Can you work these out from the model? Positions are in its coordinate system, mm. A direction names the side the tool comes from. Coordinates: 2 decimals unless noted, no trailing zeros. Loops run counter-clockwise (first coordinate to the right, second up) from the corner with the lowest first, then second, coordinate; pieces in that order, holes last.
```python
from build123d import *

# Parameters (mm, degrees)
CROQUIS1_W              = 20
CROQUIS1_H              = 72.5
CROQUIS1_R              = 1.6
SALIENTE_EXTRUIR1_DEPTH = 5
CORTAR_EXTRUIR1_DEPTH   = 2
CROQUIS3_W              = 20
CROQUIS3_H              = 8
SALIENTE_EXTRUIR2_DEPTH = 45
CROQUIS4_R              = 2.25
CROQUIS4_R_2            = 3
CORTAR_EXTRUIR2_DEPTH   = 45
CROQUIS5_W              = 15
CROQUIS5_H              = 45
CROQUIS5_R              = 1.6
SALIENTE_EXTRUIR3_DEPTH = 2
REDONDEO2_R             = 2
REDONDEO3_R             = 10


with BuildPart() as part:
    # Croquis1 → Saliente-Extruir1 (new body)
    with BuildSketch(Plane(origin=(0, 0, 0), x_dir=(1, 0, 0), z_dir=(0, 1, 0))):
        Rectangle(CROQUIS1_W, CROQUIS1_H)
        with Locations(Location((-5, 31.25, 0), (0, 0, 270))):
            Circle(CROQUIS1_R, mode=Mode.SUBTRACT)
        with Locations(Location((5, 31.25, 0), (0, 0, 270))):
            Circle(CROQUIS1_R, mode=Mode.SUBTRACT)
        with Locations(Location((-5, -31.25, 0), (0, 0, 270))):
            Circle(CROQUIS1_R, mode=Mode.SUBTRACT)
        with Locations(Location((5, -31.25, 0), (0, 0, 270))):
            Circle(CROQUIS1_R, mode=Mode.SUBTRACT)
    extrude(amount=SALIENTE_EXTRUIR1_DEPTH)

    # Croquis2 → Cortar-Extruir1 (cut)
    with BuildSketch(Plane(origin=(0, 5, 0), x_dir=(1, 0, 0), z_dir=(0, 1, 0))):
        Polygon((-2.15, 29.604551733), (-2.15, 32.895448267), (-5, 34.540896534), (-7.85, 32.895448267), (-7.85, 29.604551733), (-5, 27.959103466), align=None)
        Polygon((5, 27.959103466), (7.85, 29.604551733), (7.85, 32.895448267), (5, 34.540896534), (2.15, 32.895448267), (2.15, 29.604551733), align=None)
        Polygon((-5, -34.540896534), (-2.15, -32.895448267), (-2.15, -29.604551733), (-5, -27.959103466), (-7.85, -29.604551733), (-7.85, -32.895448267), align=None)
        Polygon((5, -27.959103466), (2.15, -29.604551733), (2.15, -32.895448267), (5, -34.540896534), (7.85, -32.895448267), (7.85, -29.604551733), align=None)
    extrude(amount=-CORTAR_EXTRUIR1_DEPTH, mode=Mode.SUBTRACT)

    # Croquis3 → Saliente-Extruir2 (add)
    with BuildSketch(Plane(origin=(0, 5, 0), x_dir=(1, 0, 0), z_dir=(0, 1, 0))):
        with Locations((0, -22.25)):
            Rectangle(CROQUIS3_W, CROQUIS3_H)
    extrude(amount=SALIENTE_EXTRUIR2_DEPTH)

    # Croquis4 → Cortar-Extruir2 (cut)
    with BuildSketch(Plane(origin=(0, 0, 18.25), x_dir=(-1, 0, 0), z_dir=(0, 0, -1))):
        with Locations((-2, 10)):
            Circle(CROQUIS4_R)
        with Locations((-2, 45)):
            Circle(CROQUIS4_R)
        with Locations((-2, 34)):
            Circle(CROQUIS4_R_2)
    extrude(amount=-CORTAR_EXTRUIR2_DEPTH, mode=Mode.SUBTRACT)

    # Croquis5 → Saliente-Extruir3 (add)
    with BuildSketch(Plane.ZY.offset(10)):
        with Locations((10.75, 27.5)):
            Rectangle(CROQUIS5_W, CROQUIS5_H)
        with Locations((13.15, 42)):
            Circle(CROQUIS5_R, mode=Mode.SUBTRACT)
        with Locations((13.15, 10)):
            Circle(CROQUIS5_R, mode=Mode.SUBTRACT)
    extrude(amount=-SALIENTE_EXTRUIR3_DEPTH)

    # Redondeo2
    # the kernel refuses this fillet: 2 mm, written as the material it adds along each edge
    with BuildSketch(Plane(origin=(-10, 5, 26.25), x_dir=(0, 1, 0), z_dir=(1, 0, 0))) as redondeo2_piece_1_section:
        with BuildLine():
            CenterArc((REDONDEO2_R, REDONDEO2_R), REDONDEO2_R, 180, 90)
            Line((0, REDONDEO2_R), (0, 0))
            Line((0, 0), (REDONDEO2_R, 0))
        make_face()
    redondeo2_piece_1 = extrude(amount=20, mode=Mode.PRIVATE)
    redondeo2_piece_1 = split(redondeo2_piece_1, bisect_by=Plane(origin=(-7.126844401, 5.386325592, 29.187037653), z_dir=(-0.4999999999999993, 0, -0.866025403784439)), keep=Keep.TOP, mode=Mode.PRIVATE)
    redondeo2_piece_1 = split(redondeo2_piece_1, bisect_by=Plane(origin=(-8.118654127, 5.386325592, 26.158547666), z_dir=(-0.49999999999999917, 0, 0.8660254037844392)), keep=Keep.TOP, mode=Mode.PRIVATE)
    add(redondeo2_piece_1)
    with BuildSketch(Plane(origin=(-10, 5, 26.25), x_dir=(0, 1, 0), z_dir=(1, 0, 0))) as redondeo2_piece_2_section:
        with BuildLine():
            CenterArc((REDONDEO2_R, REDONDEO2_R), REDONDEO2_R, 180, 90)
            Line((0, REDONDEO2_R), (0, 0))
            Line((0, 0), (REDONDEO2_R, 0))
        make_face()
    redondeo2_piece_2 = extrude(amount=20, mode=Mode.PRIVATE)
    redondeo2_piece_2 = split(redondeo2_piece_2, bisect_by=Plane(origin=(-4.392913505, 5.539408931, 27.608601914), z_dir=(-0.4999999999999993, 0, -0.866025403784439)), keep=Keep.TOP, mode=Mode.PRIVATE)
    redondeo2_piece_2 = split(redondeo2_piece_2, bisect_by=Plane(origin=(-5.607086495, 5.539408931, 27.608601914), z_dir=(0.49999999999999917, 0, -0.8660254037844392)), keep=Keep.TOP, mode=Mode.PRIVATE)
    add(redondeo2_piece_2)
    with BuildSketch(Plane(origin=(-10, 5, 26.25), x_dir=(0, 1, 0), z_dir=(1, 0, 0))) as redondeo2_piece_3_section:
        with BuildLine():
            CenterArc((REDONDEO2_R, REDONDEO2_R), REDONDEO2_R, 180, 90)
            Line((0, REDONDEO2_R), (0, 0))
            Line((0, 0), (REDONDEO2_R, 0))
        make_face()
    redondeo2_piece_3 = extrude(amount=20, mode=Mode.PRIVATE)
    redondeo2_piece_3 = split(redondeo2_piece_3, bisect_by=Plane(origin=(0.754095137, 5.386325592, 25.50772915), z_dir=(-0.4999999999999997, 0, 0.8660254037844388)), keep=Keep.TOP, mode=Mode.PRIVATE)
    redondeo2_piece_3 = split(redondeo2_piece_3, bisect_by=Plane(origin=(1.745904863, 5.386325592, 29.837856169), z_dir=(-0.5000000000000001, 0, -0.8660254037844386)), keep=Keep.TOP, mode=Mode.PRIVATE)
    redondeo2_piece_3 = split(redondeo2_piece_3, bisect_by=Plane(origin=(-0.754095137, 5.386325592, 25.50772915), z_dir=(0.4999999999999993, 0, 0.866025403784439)), keep=Keep.TOP, mode=Mode.PRIVATE)
    redondeo2_piece_3 = split(redondeo2_piece_3, bisect_by=Plane(origin=(-1.745904863, 5.386325592, 29.837856169), z_dir=(0.49999999999999917, 0, -0.8660254037844392)), keep=Keep.TOP, mode=Mode.PRIVATE)
    add(redondeo2_piece_3)
    with BuildSketch(Plane(origin=(-10, 5, 26.25), x_dir=(0, 1, 0), z_dir=(1, 0, 0))) as redondeo2_piece_4_section:
        with BuildLine():
            CenterArc((REDONDEO2_R, REDONDEO2_R), REDONDEO2_R, 180, 90)
            Line((0, REDONDEO2_R), (0, 0))
            Line((0, 0), (REDONDEO2_R, 0))
        make_face()
    redondeo2_piece_4 = extrude(amount=20, mode=Mode.PRIVATE)
    redondeo2_piece_4 = split(redondeo2_piece_4, bisect_by=Plane(origin=(4.392913505, 5.539408931, 27.608601914), z_dir=(0.4999999999999997, 0, -0.8660254037844388)), keep=Keep.TOP, mode=Mode.PRIVATE)
    redondeo2_piece_4 = split(redondeo2_piece_4, bisect_by=Plane(origin=(5.607086495, 5.539408931, 27.608601914), z_dir=(-0.5000000000000001, 0, -0.8660254037844386)), keep=Keep.TOP, mode=Mode.PRIVATE)
    add(redondeo2_piece_4)
    with BuildSketch(Plane(origin=(-10, 5, 26.25), x_dir=(0, 1, 0), z_dir=(1, 0, 0))) as redondeo2_piece_5_section:
        with BuildLine():
            CenterArc((REDONDEO2_R, REDONDEO2_R), REDONDEO2_R, 180, 90)
            Line((0, REDONDEO2_R), (0, 0))
            Line((0, 0), (REDONDEO2_R, 0))
        make_face()
    redondeo2_piece_5 = extrude(amount=20, mode=Mode.PRIVATE)
    redondeo2_piece_5 = split(redondeo2_piece_5, bisect_by=Plane(origin=(7.126844401, 5.386325592, 29.187037653), z_dir=(0.4999999999999997, 0, -0.8660254037844388)), keep=Keep.TOP, mode=Mode.PRIVATE)
    redondeo2_piece_5 = split(redondeo2_piece_5, bisect_by=Plane(origin=(8.118654127, 5.386325592, 26.158547666), z_dir=(0.5000000000000001, 0, 0.8660254037844386)), keep=Keep.TOP, mode=Mode.PRIVATE)
    add(redondeo2_piece_5)
    # the kernel refuses this fillet: 2 mm, written as the material it takes off along each edge
    with BuildSketch(Plane(origin=(-15, 50, 26.25), x_dir=(0, -1, 0), z_dir=(1, 0, 0))) as redondeo2_2_piece_1:
        with BuildLine():
            CenterArc((REDONDEO2_R, REDONDEO2_R), REDONDEO2_R, 180, 90)
            Line((0, REDONDEO2_R), (0, 0))
            Line((0, 0), (REDONDEO2_R, 0))
        make_face()
    extrude(amount=30, mode=Mode.SUBTRACT)
    with BuildSketch(Plane(origin=(-15, 50, 3.25), x_dir=(0, 0, 1), z_dir=(1, 0, 0))) as redondeo2_2_piece_2:
        with BuildLine():
            CenterArc((REDONDEO2_R, REDONDEO2_R), REDONDEO2_R, 180, 90)
            Line((0, REDONDEO2_R), (0, 0))
            Line((0, 0), (REDONDEO2_R, 0))
        make_face()
    extrude(amount=12, mode=Mode.SUBTRACT)
    with BuildSketch(Plane(origin=(-10, -5, -36.25), x_dir=(1, 0, 0), z_dir=(0, 1, 0)), Plane(origin=(10, -5, 36.25), x_dir=(-1, 0, 0), z_dir=(0, 1, 0))) as redondeo2_2_piece_3:
        with BuildLine():
            CenterArc((REDONDEO2_R, -REDONDEO2_R), REDONDEO2_R, 90, 90)
            Line((0, -REDONDEO2_R), (0, 0))
            Line((0, 0), (REDONDEO2_R, 0))
        make_face()
    extrude(amount=15, mode=Mode.SUBTRACT)
    with BuildSketch(Plane(origin=(10, -5, -36.25), x_dir=(-1, 0, 0), z_dir=(0, 1, 0)), Plane(origin=(-10, -5, 36.25), x_dir=(1, 0, 0), z_dir=(0, 1, 0))) as redondeo2_2_piece_4:
        with BuildLine():
            CenterArc((REDONDEO2_R, REDONDEO2_R), REDONDEO2_R, 180, 90)
            Line((0, REDONDEO2_R), (0, 0))
            Line((0, 0), (REDONDEO2_R, 0))
        make_face()
    extrude(amount=15, mode=Mode.SUBTRACT)

    # Redondeo3
    redondeo3_edges = [part.edges().sort_by_distance(p)[0] for p in [
        (-9, 5, 3.25),
    ]]
    fillet(redondeo3_edges, radius=REDONDEO3_R)


solid = part.part
```
Item 1: I need wall thicknesses on line 1 along Y through (x, z) = (-9.4, 13.15); line 2 along Y through (x, z) = (2, 21.25); line 3 along X through (y, z) = (3.5, 33.5). Which ranges of each line are inside material? Lowest first, please.
Results are:
line 1: y = 0 to 8.4, 11.6 to 40.4, 43.6 to 50
line 2: y = 0 to 7.75, 12.25 to 31, 37 to 42.75, 47.25 to 50
line 3: x = -10 to -6.8, -3.2 to 3.2, 6.8 to 10
Item 2: Suppose I cut it at D-D, the plane y = 10. Please give me the cut outline in (x, z).
Results are:
outline: (-10, 1.91) - (-8, 1.91) - (-8, 11.55) - (-10, 11.55) - close; (-10, 14.75) - (-8, 14.75) - (-8, 18.25) - (-0.25, 18.25) - (-0.25, 26.25) - (-10, 26.25) - close; (4.25, 18.25) - (10, 18.25) - (10, 26.25) - (4.25, 26.25) - close
Item 3: Suppose I cut it at A-A, the plane z = 23. Please give me the cut outline in (x, y).
Results are:
outline: (-10, 0) - (10, 0) - (10, 50) - (-10, 50) - close; hole circle Ø6 at (2, 34); hole circle Ø4.5 at (2, 10); hole circle Ø4.5 at (2, 45)
Item 4: Suppose I cut it at B-B, the plane y = 45. Please give me the cut outline in (x, z).
Results are:
outline: (-10, 3.25) - (-8, 3.25) - (-8, 18.25) - (-0.25, 18.25) - (-0.25, 26.25) - (-10, 26.25) - close; (4.25, 18.25) - (10, 18.25) - (10, 26.25) - (4.25, 26.25) - close
Item 5: I'm going to push flat-ended pins straight in: P1, Ø5, axis at x = 2, y = 34, coming from the -Z side; P2, Ø10, axis at x = -1.5, y = 14.5, coming from the +Z side; P3, Ø1.5, axis at x = -3.5, y = 35, coming from the -Z side; P4, Ø1.7, axis at x = 5.5, z = 30, coming from the +Y side. Where does each tip first touch, or does it pass through?
Results are:
P1: passes through
P2: stops at z = 26.25
P3: stops at z = 18.25
P4: stops at y = 3
Item 6: Suppose I cut it at C-C, the plane z = -31.25. Please give me the cut outline in (x, y).
Results are:
outline: (-10, 0) - (-6.6, 0) - (-6.6, 3) - (-7.85, 3) - (-7.85, 5) - (-10, 5) - close; (-3.4, 0) - (3.4, 0) - (3.4, 3) - (2.15, 3) - (2.15, 5) - (-2.15, 5) - (-2.15, 3) - (-3.4, 3) - close; (6.6, 0) - (10, 0) - (10, 5) - (7.85, 5) - (7.85, 3) - (6.6, 3) - close
Item 7: We'd pull the mould along X, two halves only. Please class faces 4 (the face through (-4.93, 1.48, 29.65)), 5 (the face through (-9.43, 2.46, 35.65)), 6 (the face through (-6.405, 4.014, -33.73)), 7 (the face through (-0.14, 49.43, 25.65)): +X half, -X half, draft (parallel to the pull), parting line (faces both ways), or undercut.
Results are:
face 4: undercut
face 5: -X half
face 6: undercut
face 7: draft
Item 8: On a 3-axis mill with a long thin cutter (end or side, diameter ignored), from which of +Z, -Z, +X, -X, +Y, -Y can I reach the whole of each face in a straight line? I mean faces 1 (the face through (6.405, 4.014, 33.73)), 2 (the face through (0.79, 11.897, 22.194)), 3 (the face through (-8, 28, 11)). Say none if no direction works.
Results are:
face 1: +Y
face 2: +Z, -Z
face 3: -Z, +X, +Y
